from build123d import *

# Parameters (mm, degrees)
ESQUISSE1_W                  = 57
ESQUISSE1_H                  = 57
ESQUISSE1_W_2                = 50.5
ESQUISSE1_H_2                = 50.5
BOSS_EXTRU_1_DEPTH           = 75
ENL_V_MAT_EXTRU_1_DEPTH      = 99.418748214
ENL_V_MAT_EXTRU_1_DEPTH_BACK = 99.418748214
ESQUISSE2_R                  = 4
ESQUISSE3_W                  = 52
ESQUISSE3_H                  = 34
BOSS_EXTRU_2_DEPTH           = 3
BOSS_EXTRU_3_START           = -23
ESQUISSE4_R                  = 2.5
BOSS_EXTRU_3_DEPTH           = 3
CONG_1_R                     = 5
BOSS_EXTRU_4_START           = -6.5
BOSS_EXTRU_4_DEPTH           = 3
ESQUISSE9_W                  = 13
ESQUISSE9_H                  = 13
ESQUISSE9_R                  = 1.5
BOSS_EXTRU_5_DEPTH           = 3
CONG_2_R                     = 10


with BuildPart() as part:
    # Esquisse1 → Boss.-Extru.1 (new body)
    with BuildSketch(Plane.XY):
        Rectangle(ESQUISSE1_W, ESQUISSE1_H)
        Rectangle(ESQUISSE1_W_2, ESQUISSE1_H_2, mode=Mode.SUBTRACT)
    extrude(amount=BOSS_EXTRU_1_DEPTH)

    # Esquisse2 → Enlèv. mat.-Extru.1 (cut, two sides: drawn at the far end of the back side and taken through both)
    with BuildSketch(Plane.XZ.offset(28.5).offset(-ENL_V_MAT_EXTRU_1_DEPTH_BACK)):
        with Locations(Location((0, 37.5, 0), (0, 0, 270))):
            Circle(ESQUISSE2_R)
    extrude(amount=ENL_V_MAT_EXTRU_1_DEPTH + ENL_V_MAT_EXTRU_1_DEPTH_BACK, mode=Mode.SUBTRACT)

    # Esquisse3 → Boss.-Extru.2 (add)
    with BuildSketch(Plane(origin=(0, 0, 0), x_dir=(-1, 0, 0), z_dir=(0, 0, -1))):
        with Locations((0, -45.5)):
            Rectangle(ESQUISSE3_W, ESQUISSE3_H)
    extrude(amount=-BOSS_EXTRU_2_DEPTH)

    # Esquisse4 → Boss.-Extru.3 (add)
    with BuildSketch(Plane.XZ.offset(62.5).offset(BOSS_EXTRU_3_START)):
        with BuildLine():
            Line((-22.5, 3), (-22.5, 37.5))
            Line((-22.5, 37.5), (-5, 37.5))
            ThreePointArc((-5, 37.5), (0, 32.5), (5, 37.5))
            Line((5, 37.5), (22.5, 37.5))
            Line((22.5, 37.5), (22.5, 3))
            Line((22.5, 3), (-22.5, 3))
        make_face()
        with Locations(Location((-17.5, 30, 0), (0, 0, 270))):
            Circle(ESQUISSE4_R, mode=Mode.SUBTRACT)
        with Locations(Location((17.5, 30, 0), (0, 0, 90))):
            Circle(ESQUISSE4_R, mode=Mode.SUBTRACT)
    extrude(amount=BOSS_EXTRU_3_DEPTH)

    # Congé1
    cong_1_edges = [part.edges().sort_by_distance(p)[0] for p in [
        (-22.5, -41, 37.5),
        (22.5, -41, 37.5),
    ]]
    fillet(cong_1_edges, radius=CONG_1_R)

    # Esquisse8 → Boss.-Extru.4 (add)
    with BuildSketch(Plane.ZY.offset(22.5).offset(BOSS_EXTRU_4_START)):
        Polygon((3, -28.5), (8, -28.5), (20, -39.5), (3, -39.5), align=None)
    boss_extru_4 = extrude(amount=BOSS_EXTRU_4_DEPTH)

    # Symétrie1: Boss.-Extru.4 across plane
    add(boss_extru_4.mirror(Plane(origin=(0, 0, 0), x_dir=(0, 0, 1), z_dir=(1, 0, 0))))

    # Esquisse9 → Boss.-Extru.5 (add)
    # profile 1 of 4: a face of its own
    with BuildSketch(Plane(origin=(0, 0, 0), x_dir=(-1, 0, 0), z_dir=(0, 0, -1))):
        with Locations((-31.819805153, 31.819805153)):
            Rectangle(ESQUISSE9_W, ESQUISSE9_H)
        with Locations((-31.819805153, 31.819805153)):
            Circle(ESQUISSE9_R, mode=Mode.SUBTRACT)
    # profile 2 of 4: a face of its own
    with BuildSketch(Plane(origin=(0, 0, 0), x_dir=(-1, 0, 0), z_dir=(0, 0, -1))):
        with Locations((31.819805153, 31.819805153)):
            Rectangle(ESQUISSE9_W, ESQUISSE9_H)
        with Locations((31.819805153, 31.819805153)):
            Circle(ESQUISSE9_R, mode=Mode.SUBTRACT)
    # profile 3 of 4: a face of its own
    with BuildSketch(Plane(origin=(0, 0, 0), x_dir=(-1, 0, 0), z_dir=(0, 0, -1))):
        with Locations((31.819805153, -31.819805153)):
            Rectangle(ESQUISSE9_W, ESQUISSE9_H)
        with Locations((31.819805153, -31.819805153)):
            Circle(ESQUISSE9_R, mode=Mode.SUBTRACT)
    # profile 4 of 4: a face of its own
    with BuildSketch(Plane(origin=(0, 0, 0), x_dir=(-1, 0, 0), z_dir=(0, 0, -1))):
        with Locations((-31.819805153, -31.819805153)):
            Rectangle(ESQUISSE9_W, ESQUISSE9_H)
        with Locations((-31.819805153, -31.819805153)):
            Circle(ESQUISSE9_R, mode=Mode.SUBTRACT)
    extrude(amount=-BOSS_EXTRU_5_DEPTH)

    # Congé2
    # the kernel refuses this fillet: 10 mm, written as the material it takes off along each edge
    with BuildSketch(Plane(origin=(-38.319805153, -38.319805153, -25), x_dir=(0, 1, 0), z_dir=(0, 0, 1)), Plane(origin=(38.319805153, -38.319805153, -25), x_dir=(-1, 0, 0), z_dir=(0, 0, 1)), Plane(origin=(38.319805153, 38.319805153, -25), x_dir=(0, -1, 0), z_dir=(0, 0, 1)), Plane(origin=(-38.319805153, 38.319805153, -25), x_dir=(1, 0, 0), z_dir=(0, 0, 1))) as cong_2_piece_1:
        with BuildLine():
            CenterArc((CONG_2_R, -CONG_2_R), CONG_2_R, 90, 90)
            Line((0, -CONG_2_R), (-CONG_2_R * 0.02, -CONG_2_R))
            Line((-CONG_2_R * 0.02, -CONG_2_R), (-CONG_2_R * 0.02, CONG_2_R * 0.02))
            Line((-CONG_2_R * 0.02, CONG_2_R * 0.02), (CONG_2_R, CONG_2_R * 0.02))
            Line((CONG_2_R, CONG_2_R * 0.02), (CONG_2_R, 0))
        make_face()
    extrude(amount=53, mode=Mode.SUBTRACT)
    with BuildSketch(Plane(origin=(-38.319805153, -25.319805153, -24.995940898), x_dir=(1, 0, 0), z_dir=(0, 0, 1)), Plane(origin=(38.319805153, 25.319805153, -24.995940898), x_dir=(-1, 0, 0), z_dir=(0, 0, 1)), Plane(origin=(-25.319805153, 38.319805153, -24.995940898), x_dir=(0, -1, 0), z_dir=(0, 0, 1))) as cong_2_piece_2:
        with BuildLine():
            CenterArc((10, -9.998376359), CONG_2_R, 91.032496301, 88.967503699)
            Line((0, -9.998376359), (-0.2, -9.998376359))
            Line((-0.2, -9.998376359), (-0.2, 0))
            Line((-0.2, 0), (0, 0.2))
            ThreePointArc((0, 0.2), (4.909902577, 0.2), (9.816201256, 0.199967527))
            Line((9.816201256, 0.199967527), (9.819805153, 0))
        make_face()
    extrude(amount=52.991881795, mode=Mode.SUBTRACT)
    with BuildSketch(Plane(origin=(38.319805153, -25.319805153, -24.995940898), x_dir=(0, -1, 0), z_dir=(0, 0, 1)), Plane(origin=(25.319805153, 38.319805153, -24.995940898), x_dir=(1, 0, 0), z_dir=(0, 0, 1)), Plane(origin=(-38.319805153, 25.319805153, -24.995940898), x_dir=(0, 1, 0), z_dir=(0, 0, 1))) as cong_2_piece_3:
        with BuildLine():
            CenterArc((9.998376359, -10), CONG_2_R, 90, 88.967503699)
            Line((0, -9.819805153), (-0.199967527, -9.816201256))
            ThreePointArc((-0.199967527, -9.816201256), (-0.2, -4.909902577), (-0.2, 0))
            Line((-0.2, 0), (0, 0.2))
            Line((0, 0.2), (9.998376359, 0.2))
            Line((9.998376359, 0.2), (9.998376359, 0))
        make_face()
    extrude(amount=52.991881795, mode=Mode.SUBTRACT)


solid = part.part
Model file for the job. Use its own axes, mm. A direction names the side the tool comes from. Give positions to 0.01 mm unless a question says otherwise; leave off trailing zeros. Loops run counter-clockwise (first coordinate to the right, second up) from the corner with the lowest first, then second, coordinate; pieces in that order, holes last.
Item 1: Slice it at D-D (z = 46.5). Write the cut outline in (x, y), plus the area to 3 significant figures.
Check values:
outline: (-28.5, -28.5) - (28.5, -28.5) - (28.5, 28.5) - (-28.5, 28.5) - close; hole (-25.25, -25.25) - (25.25, -25.25) - (25.25, 25.25) - (-25.25, 25.25) - close
area: 699 mm2
Item 2: Slice it at A-A (z = 30). Write the cut outline in (x, y), plus the area to 3 significant figures.
Check values:
outline: (-28.5, -28.5) - (28.5, -28.5) - (28.5, 28.5) - (-28.5, 28.5) - close; (-22.5, -42.5) - (-20, -42.5) - (-20, -39.5) - (-22.5, -39.5) - close; (-15, -42.5) - (15, -42.5) - (15, -39.5) - (-15, -39.5) - close; (20, -42.5) - (22.5, -42.5) - (22.5, -39.5) - (20, -39.5) - close; hole (-25.25, -25.25) - (25.25, -25.25) - (25.25, 25.25) - (-25.25, 25.25) - close
area: 804 mm2
Item 3: Slice it at C-C (x = 10). Write the cut outline in (y, z).
Check values:
outline: (-62.5, 0) - (-25.25, 0) - (-25.25, 75) - (-28.5, 75) - (-28.5, 3) - (-39.5, 3) - (-39.5, 37.5) - (-42.5, 37.5) - (-42.5, 3) - (-62.5, 3) - close; (25.25, 0) - (28.5, 0) - (28.5, 75) - (25.25, 75) - close
Item 4: Drop flat-ended pins along their axis: P1, Ø1.8, axis at x = -31.82, y = 31.82, coming from the +Z side; P2, Ø12, axis at y = -34, z = 7.5, coming from the +X side; P3, Ø0.9, axis at x = 10.5, y = -41, coming from the +Z side; P4, Ø4, axis at y = -11.5, z = 58, coming from the +X side. Give the stop position or say it passes through.
Check values:
P1: passes through
P2: stops at x = 37.69
P3: stops at z = 37.5
P4: stops at x = 28.5
Item 5: Drill centre lines: line 1 along X through (y, z) = (-40, 30); line 2 along Y through (x, z) = (19.5, 49). Where is each one in solid material? Low to high.
Check values:
line 1: x = -22.5 to -20, -15 to 15, 20 to 22.5
line 2: y = -28.5 to -25.25, 25.25 to 28.5
Item 6: Slice it at B-B (y = 17.5). Write the cut outline in (x, z).
Check values:
outline: (-28.5, 0) - (-25.25, 0) - (-25.25, 75) - (-28.5, 75) - close; (25.25, 0) - (28.5, 0) - (28.5, 75) - (25.25, 75) - close
Item 7: Mould opens along Y. For faces 1 (the face through (-26, -51, 1)), 2 (the face through (0, -62.5, 1)), 3 (the face through (-7, -28.5, 38)) say: +Y half, -Y half, draft (parallel to the pull), parting line (faces both ways), or undercut.
Check values:
face 1: draft
face 2: -Y half
face 3: undercut
Item 8: Which spindle directions (+Z, -Z, +X, -X, +Y, -Y) get a long thin tool onto all of the face, cutting with end or side? Do faces 4 (the face through (26, -51, 1)), 5 (the face through (19, -35, 10)), 6 (the face through (-34.03, -27.11, 1.48)). Say none if no direction does.
Check values:
face 4: +Z, -Z, +X, -Y
face 5: +Z, +X
face 6: +Z, -Z, -X
